Check sheet for the modelled part. Datum: model origin and axes. Units: mm. Face numbers are marked on the shaded views. Coordinates: 2 decimals unless noted, no trailing zeros. Write each question's results on one line, items separated by ' | '. Start each with the question number.
1. Draft check along Y on the marked faces 1 and 2. Enter one of: released by +Y, released by -Y, zero draft, split by the parting line, or undercut.
2. Thickness scan on line 1 (Y direction, x = 0, z = -45); line 2 (Y direction, x = -5.5, z = -14). Record the ranges inside material, lowest first. Write a range as [from, to].
3. Gauge pin test, flat ends, axial feed: P1, Ø4, axis at x = 8.5, y = 3.5, coming from the -Z side; P2, Ø1, axis at x = 6, z = -41, coming from the +Y side; P3, Ø10, axis at x = -1, y = 12.5, coming from the -Z side; P4, Ø5, axis at y = 11, z = -7, coming from the +X side. Record the tip position at first contact, or that the pin passes through.
```python
from build123d import *

# Parameters (mm, degrees)
F3_DEPTH  = 5
F5_DEPTH  = 15
F6_W      = 2
F6_H      = 3
F7_DEPTH  = 20.5
F8_W      = 3
F8_H      = 1
F9_DEPTH  = 17.5068136575
F10_R     = 0.3
F11_R     = 0.1
F12_R     = 0.1
F13_W     = 100
F13_H     = 100
F14_DEPTH = 62.0010001


with BuildPart() as f2:
    # F1 (on Front) → F2 (revolve)
    with BuildSketch(Plane.XZ):
        with BuildLine():
            Line((-2, 62), (-10, 62))
            add(Edge.make_bspline(
                [(-10, 62), (-11.8174263966, 57.1809415466), (-15.8594861297, 46.4373198499), (-18.6273544316, 24.5459471202), (-15.0414654734, -19.3469968059), (-5.4834802074, -38.7438846901), (-1.25, -47.0509425635)],
                knots=[0, 0, 0, 0, 0.1886807773, 0.4119593541, 0.7294893705, 0.9757699691, 0.9757699691, 0.9757699691, 0.9757699691], degree=3))
            Line((-1.25, -47.0509425635), (-1.25, -43.0509425635))
            Line((-1.25, -43.0509425635), (-1.75, -43.0509425635))
            Line((-1.75, -43.0509425635), (-1.75, -19.5))
            Line((-1.75, -19.5), (0, -19.5))
            Line((0, -19.5), (0, 47))
            Line((0, 47), (0, 50))
            Line((0, 50), (-2, 50))
            Line((-2, 50), (-2, 62))
        make_face()
    revolve(axis=Axis((0, 0, 54.5), (0, 0, 1)))

    # F0 (on Front) → F3 (cut, symmetric)
    with BuildSketch(Plane.XZ):
        Polygon((-10.75, -19.5), (10.75, -19.5), (10.75, 44.5), (9, 44.5), (9, 50.5), (-9, 50.5), (-9, 44.5), (-10.75, 44.5), align=None)
    extrude(amount=F3_DEPTH, both=True, mode=Mode.SUBTRACT)

    # F4 (on face) → F5 (cut)
    with BuildSketch(Plane.XY.offset(62)):
        Polygon((1.2421649551, -1.9468845774), (2.3071339798, 0.1023041181), (1.0649690247, 2.0491886955), (-1.2421649551, 1.9468845774), (-2.3071339798, -0.1023041181), (-1.0649690247, -2.0491886955), align=None)
    extrude(amount=-F5_DEPTH, mode=Mode.SUBTRACT)

    # F6 (on Right) → F7 (cut, symmetric)
    with BuildSketch(Plane.YZ):
        with Locations((-0.8976958819, 48.5)):
            Rectangle(F6_W, F6_H)
    extrude(amount=F7_DEPTH, both=True, mode=Mode.SUBTRACT)

    # F8 (on Front) → F9 (cut, through all)
    with BuildSketch(Plane.XZ):
        with Locations((0, 41.5)):
            Rectangle(F8_W, F8_H)
    extrude(amount=F9_DEPTH, mode=Mode.SUBTRACT)

    # F10
    f10_edges = [f2.edges().sort_by_distance(p)[0] for p in [
        (1.25, 0, -47.050943),
    ]]
    fillet(f10_edges, radius=F10_R)

    # F11
    f11_edges = [f2.edges().sort_by_distance(p)[0] for p in [
        (1.25, 0, -43.050943),
    ]]
    fillet(f11_edges, radius=F11_R)

    # F12
    f12_edges = [f2.edges().sort_by_distance(p)[0] for p in [
        (1.75, 0, -43.050943),
    ]]
    fillet(f12_edges, radius=F12_R)

    # F13 (on Top) → F14 (cut, through all)
    with BuildSketch(Plane.XY):
        Rectangle(F13_W, F13_H)
    extrude(amount=F14_DEPTH, mode=Mode.SUBTRACT)


solid = f2.part
```
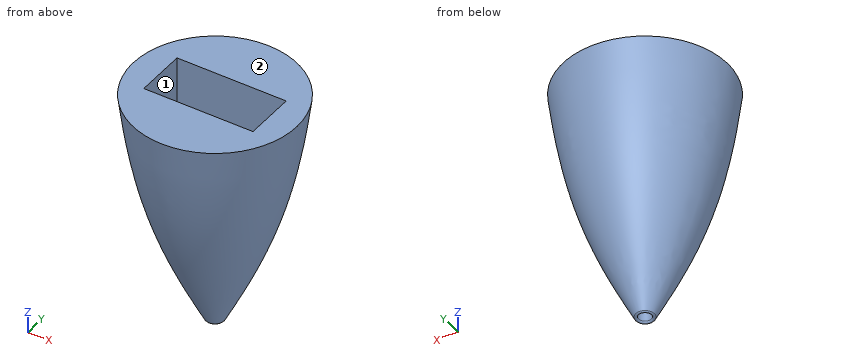
Established:
1) face 1: undercut | face 2: zero draft
2) line 1: [-2.29, -1.25], [1.25, 2.29] | line 2: [-12.66, -5], [5, 12.66]
3) P1: z = -34.67 | P2: through | P3: z = -33.86 | P4: x = 12.53
